from build123d import *

# Parameters (mm, degrees)
SKETCH_1_W           = 250
SKETCH_1_H           = 65
SKETCH_1_R           = 2.5
EXTRUDE_1_DEPTH      = 3
FILLET_1_R           = 3
CUT_EXTRUDE_3_DEPTH  = 4
FILLET_2_R           = 3
SKETCH_6_W           = 30
SKETCH_6_H           = 65
CUT_EXTRUDE_4_DEPTH  = 5
CUT_EXTRUDE_7_DEPTH  = 5
FILLET_3_R           = 5
SKETCH_8_R           = 2.5
EXTRUDE_2_DEPTH      = 3
SKETCH_10_R          = 2.5
CUT_EXTRUDE_8_DEPTH  = 3
SKETCH_13_R          = 2.5
EXTRUDE_3_DEPTH      = 3
SKETCH_15_R          = 2.5
EXTRUDE_4_DEPTH      = 3
SKETCH_18_R          = 2.5
CUT_EXTRUDE_11_DEPTH = 4
SKETCH_20_R          = 2.5
CUT_EXTRUDE_12_DEPTH = 10
SKETCH_21_R          = 2.6
CUT_EXTRUDE_13_DEPTH = 4


with BuildPart() as part:
    # 草图1 → 凸台-拉伸1 (new body)
    with BuildSketch(Plane.XY):
        Rectangle(SKETCH_1_W, SKETCH_1_H)
        with Locations((-70, 16)):
            Circle(SKETCH_1_R, mode=Mode.SUBTRACT)
        with Locations((-70, -16)):
            Circle(SKETCH_1_R, mode=Mode.SUBTRACT)
        with Locations((70, -16)):
            Circle(SKETCH_1_R, mode=Mode.SUBTRACT)
        with Locations((70, 16)):
            Circle(SKETCH_1_R, mode=Mode.SUBTRACT)
        with Locations((0, 16)):
            Circle(SKETCH_1_R, mode=Mode.SUBTRACT)
        with Locations((0, -16)):
            Circle(SKETCH_1_R, mode=Mode.SUBTRACT)
    extrude(amount=EXTRUDE_1_DEPTH)

    # 圆角1
    fillet_1_edges = [part.edges().sort_by_distance(p)[0] for p in [
        (125, -32.5, 1.5),
        (-125, -32.5, 1.5),
        (-125, 32.5, 1.5),
        (125, 32.5, 1.5),
    ]]
    fillet(fillet_1_edges, radius=FILLET_1_R)

    # 草图4 → 切除-拉伸3 (cut, through all)
    with BuildSketch(Plane(origin=(0, 0, 0), x_dir=(-1, 0, 0), z_dir=(0, 0, -1))):
        with BuildLine():
            Line((-113.82, 32.5), (-122, 32.5))
            ThreePointArc((-122, 32.5), (-124.121320344, 31.621320344), (-125, 29.5))
            Line((-125, 29.5), (-125, -29.5))
            ThreePointArc((-125, -29.5), (-124.121320344, -31.621320344), (-122, -32.5))
            Line((-122, -32.5), (-113.82, -32.5))
            Line((-113.82, -32.5), (-113.82, 32.5))
        make_face()
    extrude(amount=-CUT_EXTRUDE_3_DEPTH, mode=Mode.SUBTRACT)

    # 圆角2
    fillet_2_edges = [part.edges().sort_by_distance(p)[0] for p in [
        (113.82, 32.5, 1.5),
        (113.82, -32.5, 1.5),
    ]]
    fillet(fillet_2_edges, radius=FILLET_2_R)

    # 草图6 → 切除-拉伸4 (cut)
    with BuildSketch(Plane.XY.offset(3)):
        with Locations((-110, 0)):
            Rectangle(SKETCH_6_W, SKETCH_6_H)
    extrude(amount=-CUT_EXTRUDE_4_DEPTH, mode=Mode.SUBTRACT)

    # 草图7 → 切除-拉伸7 (cut)
    with BuildSketch(Plane.XY.offset(3)):
        Polygon((113.82, -32.860309594), (113.82, 33.556993736), (94.996170136, 32.5), (94.996170136, -32.5), align=None)
    extrude(amount=-CUT_EXTRUDE_7_DEPTH, mode=Mode.SUBTRACT)

    # 圆角3
    fillet_3_edges = [part.edges().sort_by_distance(p)[0] for p in [
        (-95, 32.5, 1.5),
        (-95, -32.5, 1.5),
        (94.996170136, -32.5, 1.5),
        (94.996170136, 32.5, 1.5),
    ]]
    fillet(fillet_3_edges, radius=FILLET_3_R)

    # 草图8 → 凸台-拉伸2 (add)
    with BuildSketch(Plane(origin=(0, 0, 0), x_dir=(-1, 0, 0), z_dir=(0, 0, -1))):
        with Locations((70, 16)):
            Circle(SKETCH_8_R)
        with Locations((70, -16)):
            Circle(SKETCH_8_R)
        with Locations((-70, 16)):
            Circle(SKETCH_8_R)
        with Locations((-70, -16)):
            Circle(SKETCH_8_R)
    extrude(amount=-EXTRUDE_2_DEPTH)

    # 草图10 → 切除-拉伸8 (cut)
    with BuildSketch(Plane(origin=(0, 0, 0), x_dir=(-1, 0, 0), z_dir=(0, 0, -1))):
        with Locations((-60.563944815, 16.029236842)):
            Circle(SKETCH_10_R)
        with Locations((-60.563944815, -15.970763158)):
            Circle(SKETCH_10_R)
        with Locations((62.89412836, 16.029236842)):
            Circle(SKETCH_10_R)
        with Locations((62.89412836, -15.970763158)):
            Circle(SKETCH_10_R)
    extrude(amount=-CUT_EXTRUDE_8_DEPTH, mode=Mode.SUBTRACT)

    # 草图13 → 凸台-拉伸3 (add)
    with BuildSketch(Plane(origin=(0, 0, 0), x_dir=(-1, 0, 0), z_dir=(0, 0, -1))):
        with Locations((62.89412836, 16.029236842)):
            Circle(SKETCH_13_R)
        with Locations((62.89412836, -15.970763158)):
            Circle(SKETCH_13_R)
    extrude(amount=-EXTRUDE_3_DEPTH)

    # 草图15 → 凸台-拉伸4 (add)
    with BuildSketch(Plane(origin=(0, 0, 0), x_dir=(-1, 0, 0), z_dir=(0, 0, -1))):
        with Locations((62.89412836, 16.029236843)):
            Circle(SKETCH_15_R)
        with Locations((62.89412836, -15.970763157)):
            Circle(SKETCH_15_R)
    extrude(amount=-EXTRUDE_4_DEPTH)

    # 草图18 → 切除-拉伸11 (cut, through all)
    with BuildSketch(Plane(origin=(0, 0, 0), x_dir=(-1, 0, 0), z_dir=(0, 0, -1))):
        with Locations((-84.996170136, 27.5)):
            Circle(SKETCH_18_R)
        with Locations((-84.996170136, -27.5)):
            Circle(SKETCH_18_R)
    cut_extrude_11 = extrude(amount=-CUT_EXTRUDE_11_DEPTH, mode=Mode.SUBTRACT)

    # 镜向1: 切除-拉伸11 across plane
    add(cut_extrude_11.mirror(Plane(origin=(-0.001914932, 0, 0), x_dir=(0, 0, 1), z_dir=(1, 0, 0))), mode=Mode.SUBTRACT)

    # 草图20 → 切除-拉伸12 (cut)
    with BuildSketch(Plane(origin=(0, 0, 0), x_dir=(-1, 0, 0), z_dir=(0, 0, -1))):
        with Locations((85, 0)):
            Circle(SKETCH_20_R)
        with Locations((-84.996170136, 0)):
            Circle(SKETCH_20_R)
    extrude(amount=-CUT_EXTRUDE_12_DEPTH, mode=Mode.SUBTRACT)

    # 草图21 → 切除-拉伸13 (cut, through all)
    with BuildSketch(Plane(origin=(0, 0, 0), x_dir=(-1, 0, 0), z_dir=(0, 0, -1))):
        with Locations((-84.996170136, 27.5)):
            Circle(SKETCH_21_R)
        with Locations((-60.563944815, 16.029236842)):
            Circle(SKETCH_21_R)
        with Locations((-84.996170136, 0)):
            Circle(SKETCH_21_R)
        with Locations((-60.563944815, -15.970763158)):
            Circle(SKETCH_21_R)
        with Locations((-84.996170136, -27.512746042)):
            Circle(SKETCH_21_R)
        with Locations((0.001914932, 16.029236842)):
            Circle(SKETCH_21_R)
        with Locations((0.001914932, -15.970763158)):
            Circle(SKETCH_21_R)
        with Locations((85, -27.512746042)):
            Circle(SKETCH_21_R)
        with Locations((60.567774678, -15.970763158)):
            Circle(SKETCH_21_R)
        with Locations((85, 0)):
            Circle(SKETCH_21_R)
        with Locations((60.567774678, 16.029236842)):
            Circle(SKETCH_21_R)
        with Locations((85, 27.5)):
            Circle(SKETCH_21_R)
    extrude(amount=-CUT_EXTRUDE_13_DEPTH, mode=Mode.SUBTRACT)


solid = part.part
Here's how the part is built. I have some questions about the finished solid (model axes, mm). Give positions to 0.01 mm unless a question says otherwise; leave off trailing zeros. Order: outer loops, then holes, each group sorted by start corner. A loop starts at its lowest first (then second) coordinate and runs counter-clockwise, first axis right, second up. Notation, with made-up numbers: (36.5, -36) -> (94.5, -36) arc R20 ccw to (94.5, -30) -> close; hole circle Ø9 at (36.25, 12). An arc over 180 degrees is marked (long way). One line per item, written item: value. Start each with the question number.
1. We'd pull the mould along Y, two halves only. Please class faces 1 (the face through (-63.048, -15.19, 1.479)), 2 (the face through (-82.403, -27.398, 1.479)), 3 (the face through (-1, 0, 3)), 4 (the face through (93.57, -30.996, 1.479)): released by +Y, released by -Y, zero draft, split by the parting line, or undercut.
2. Imagine slicing it at C-C, the plane z = 2. Count the separate pieces of the cut face and the enclosed holes in it, plus the area to 3 significant figures.
3. Imagine slicing it at B-B, the plane x = -85. List the corners of the cut face in (y, z) for me, plus the area to 3 significant figures.
4. Will these pins go through, and if not, where does the flat tip stop? pin 1 Ø3 at (x, y) = (-60.57, -15.97) entering from -Z; pin 2 Ø8.5 at (x, y) = (60.56, -15.97) entering from -Z.
5. I need wall thicknesses on probe 1 along X at (y, z) = (-27.5, 1.7); probe 2 along Y at (x, z) = (-85, 0.7); probe 3 along X at (y, z) = (29.5, 2.4). Which ranges of each line are inside material? Lowest first, please. Write a range as from..to.
6. Imagine slicing it at A-A, the plane y = 0. List the corners of the cut face in (x, z) for me.
Values follow:
1. face 1: undercut
1. face 2: undercut
1. face 3: zero draft
1. face 4: released by -Y
2. separate pieces: 1
2. enclosed holes: 12
2. area: 12,100 mm2
3. outline: (-32.5, 0) -> (-30.11, 0) -> (-30.11, 3) -> (-32.5, 3) -> close; (-24.91, 0) -> (-2.6, 0) -> (-2.6, 3) -> (-24.91, 3) -> close; (2.6, 0) -> (24.9, 0) -> (24.9, 3) -> (2.6, 3) -> close; (30.1, 0) -> (32.5, 0) -> (32.5, 3) -> (30.1, 3) -> close
3. area: 148 mm2
4. pin 1: passes through
4. pin 2: stops at z = 0
5. probe 1: x = -95..-87.6, -82.4..82.4, 87.6..95
5. probe 2: y = -32.5..-30.11, -24.91..-2.6, 2.6..24.9, 30.1..32.5
5. probe 3: x = -94.58..-86.66, -83.34..83.33, 86.66..94.58
6. outline: (-95, 0) -> (-87.6, 0) -> (-87.6, 3) -> (-95, 3) -> close; (-82.4, 0) -> (82.4, 0) -> (82.4, 3) -> (-82.4, 3) -> close; (87.6, 0) -> (95, 0) -> (95, 3) -> (87.6, 3) -> close
